Build history of the part. All positions in model axes, mm. Give positions to 0.01 mm unless a question says otherwise; leave off trailing zeros. Order: outer loops, then holes, each group sorted by start corner. A loop starts at its lowest first (then second) coordinate and runs counter-clockwise, first axis right, second up. Notation, with made-up numbers: (30, -22) - (44, -22) arc R27 ccw to (44, 16) - close; hole circle Ø4 at (4.25, 56.5). An arc over 180 degrees is marked (long way). Use a Markdown table: item, result. Add a question column.
(1) Slice it at A-A (z = 0). Write the cut outline in (x, y).
(2) Flat gauge pin, fed straight in: pin 1 (12 mm diameter, centred on y = 4, z = -260, fed in from -X). Where does the tip first touch, or does it go through?
(3) Wall check: line 1 (Y direction, x = -6, z = -310); line 2 (X direction, y = 16.5, z = -141.5); line 3 (Y direction, x = 11.8, z = 0). Give the ranges that are in metal, low to high.
(4) Slice it at B-B (x = -1.75). Write the cut outline in (y, z), then the cut area to 3 significant figures.
(5) Slice it at C-C (z = -148). Write the cut outline in (x, y).
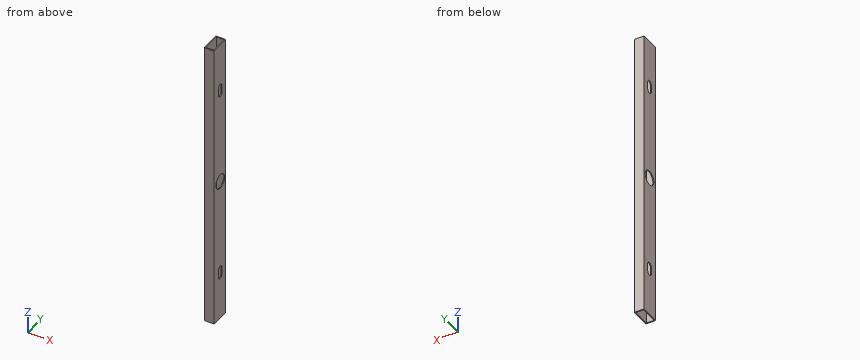
from build123d import *

# Parameters (mm, degrees)
SKETCH1_W           = 25.4
SKETCH1_H           = 50.8
SKETCH1_W_2         = 20.32
SKETCH1_H_2         = 45.72
EXTRUDE_THIN1_DEPTH = 381
SKETCH3_R           = 19.05
CUT_EXTRUDE1_DEPTH  = 383.689587002


with BuildPart() as part:
    # Sketch1 → Extrude-Thin1 (new, symmetric)
    with BuildSketch(Plane.XY):
        Rectangle(SKETCH1_W, SKETCH1_H)
        Rectangle(SKETCH1_W_2, SKETCH1_H_2, mode=Mode.SUBTRACT)
    extrude(amount=EXTRUDE_THIN1_DEPTH, both=True)

    # Sketch3 → Cut-Extrude1 (cut, through all)
    with BuildSketch(Plane(origin=(12.7, 0, 0), x_dir=(0, 0, -1), z_dir=(1, 0, 0))):
        with Locations((0, 1.524)):
            Circle(SKETCH3_R)
        with BuildLine():
            Line((244.475, 9.4615), (263.525, 9.4615))
            ThreePointArc((263.525, 9.4615), (271.4625, 1.524), (263.525, -6.4135))
            Line((263.525, -6.4135), (244.475, -6.4135))
            ThreePointArc((244.475, -6.4135), (236.5375, 1.524), (244.475, 9.4615))
        make_face()
        with BuildLine():
            Line((-244.475, 9.4615), (-263.525, 9.4615))
            ThreePointArc((-263.525, 9.4615), (-271.4625, 1.524), (-263.525, -6.4135))
            Line((-263.525, -6.4135), (-244.475, -6.4135))
            ThreePointArc((-244.475, -6.4135), (-236.5375, 1.524), (-244.475, 9.4615))
        make_face()
    extrude(amount=-CUT_EXTRUDE1_DEPTH, mode=Mode.SUBTRACT)


solid = part.part
Solution:
| question | item | result |
|---|---|---|
| 1 | outline | (-12.7, -25.4) - (12.7, -25.4) - (12.7, -17.53) - (10.16, -17.53) - (10.16, -22.86) - (-10.16, -22.86) - (-10.16, -17.53) - (-12.7, -17.53) - close; (-12.7, 20.57) - (-10.16, 20.57) - (-10.16, 22.86) - (10.16, 22.86) - (10.16, 20.57) - (12.7, 20.57) - (12.7, 25.4) - (-12.7, 25.4) - close |
| 2 | pin 1 | x = -12.7 |
| 3 | line 1 | -25.4 to -22.86, 22.86 to 25.4 |
| 3 | line 2 | -12.7 to -10.16, 10.16 to 12.7 |
| 3 | line 3 | -25.4 to -17.53, 20.57 to 25.4 |
| 4 | outline | (-25.4, -381) - (-22.86, -381) - (-22.86, 381) - (-25.4, 381) - close; (22.86, -381) - (25.4, -381) - (25.4, 381) - (22.86, 381) - close |
| 4 | area | 3,870 mm2 |
| 5 | outline | (-12.7, -25.4) - (12.7, -25.4) - (12.7, 25.4) - (-12.7, 25.4) - close; hole (-10.16, -22.86) - (10.16, -22.86) - (10.16, 22.86) - (-10.16, 22.86) - close |
